Source: CAD feature listing. Evaluate the final solid. Frame: model axes, mm. A direction names the side the tool comes from. Round coordinates to 2 decimals unless told otherwise and drop trailing zeros. Order: outer loops, then holes, each group sorted by start corner. A loop starts at its lowest first (then second) coordinate and runs counter-clockwise, first axis right, second up. Notation, with made-up numbers: (85.5, 64.25) -> (140.5, 64.25) arc R32 ccw to (140.5, 95.25) -> close; hole circle Ø10 at (24, -38). An arc over 180 degrees is marked (long way). Write item = value, one per line. Start each with the question number.
(1) Draft query along X for faces 4 (the face through (-27.25, 28, -8)), 5 (the face through (-22.25, 28.27, -4.83)), 6 (the face through (14.25, 36, 7)). Return one class per face: released by +X, released by -X, zero draft, split by the parting line, or undercut.
(2) Ray query, line 1 (Z direction, x = -24.5, y = 28.5); line 2 (Z direction, x = 24, y = 28); line 3 (Y direction, x = -11, z = -5). Return the intervals inside material, ascending.
(3) Reachability of faces 1 (the face through (-15.55, 38.75, -1.21)), 2 (the face through (-24, 28, -9)), 3 (the face through (4, 36, 9)) from +Z, -Z, +X, -X, +Y, -Y: full face, straight path, thin tool, end or side. Return the list, or none.
(4) Cut plane B-B on z = 0. Return the cut outline in (x, y).
(5) Cut plane C-C on y = 41. Return the cut outline in (x, z).
(6) Cut plane D-D on x = -15. Return the cut outline in (y, z).
(7) Cut plane A-A on x = 24.5. Return the cut outline in (y, z).
(8) Contact query for flat-ended pins moving along their axis: pin 1 Ø1 at (y, z) = (36.5, 8) entering from +X; pin 2 Ø10 at (x, z) = (6.5, 0.5) entering from +Y; pin 3 Ø3.5 at (x, z) = (25, 4) entering from -Y. Output: stop coordinate, or through.
from build123d import *

# Parameters (mm, degrees)
SKETCH1_W            = 40.5
SKETCH1_H            = 20
BOSS_EXTRUDE1_DEPTH  = 35.5
BOSS_EXTRUDE2_DEPTH  = 2
SKETCH3_R            = 6.4
BOSS_EXTRUDE3_DEPTH  = 1
SKETCH4_R            = 5.575
BOSS_EXTRUDE4_DEPTH  = 0.5
BOSS_EXTRUDE5_DEPTH  = 2.5
MIRROR2_COPY_1_DEPTH = 2.5
SKETCH6_R            = 2.5
BOSS_EXTRUDE6_DEPTH  = 5


with BuildPart() as part:
    # Sketch1 → Boss-Extrude1 (new body)
    with BuildSketch(Plane(origin=(0, 0, 0), x_dir=(1, 0, 0), z_dir=(0, 1, 0))):
        Rectangle(SKETCH1_W, SKETCH1_H)
    extrude(amount=BOSS_EXTRUDE1_DEPTH)

    # Sketch2 → Boss-Extrude2 (add)
    with BuildSketch(Plane(origin=(0, 35.5, 0), x_dir=(1, 0, 0), z_dir=(0, 1, 0))):
        with BuildLine():
            Line((-5.75, -9), (14.25, -9))
            Line((14.25, -9), (14.25, -4.8))
            ThreePointArc((14.25, -4.8), (16.65, 0), (14.25, 4.8))
            Line((14.25, 4.8), (14.25, 9))
            Line((14.25, 9), (-5.75, 9))
            ThreePointArc((-5.75, 9), (-20.108898944, 0), (-5.75, -9))
        make_face()
    extrude(amount=BOSS_EXTRUDE2_DEPTH)

    # Sketch3 → Boss-Extrude3 (add)
    with BuildSketch(Plane(origin=(0, 37.5, 0), x_dir=(1, 0, 0), z_dir=(0, 1, 0))):
        with Locations(Location((-10.108898944, 0, 0), (0, 0, 270))):
            Circle(SKETCH3_R)
    extrude(amount=BOSS_EXTRUDE3_DEPTH)

    # Sketch4 → Boss-Extrude4 (add)
    with BuildSketch(Plane(origin=(0, 38.5, 0), x_dir=(1, 0, 0), z_dir=(0, 1, 0))):
        with Locations(Location((-10.108898944, 0, 0), (0, 0, 270))):
            Circle(SKETCH4_R)
    extrude(amount=BOSS_EXTRUDE4_DEPTH)

    # Sketch5 → Boss-Extrude5 (add)
    with BuildSketch(Plane(origin=(0, 29.5, 0), x_dir=(1, 0, 0), z_dir=(0, 1, 0))):
        with BuildLine():
            Line((20.25, 9), (27.25, 9))
            Line((27.25, 9), (27.25, 6.25))
            Line((27.25, 6.25), (26.177050983, 6.25))
            ThreePointArc((26.177050983, 6.25), (22.25, 4.75), (26.177050983, 3.25))
            Line((26.177050983, 3.25), (27.25, 3.25))
            Line((27.25, 3.25), (27.25, 0))
            Line((27.25, 0), (20.25, 0))
            Line((20.25, 0), (20.25, 9))
        make_face()
    boss_extrude5 = extrude(amount=-BOSS_EXTRUDE5_DEPTH)

    # Mirror1: Boss-Extrude5 across plane
    add(boss_extrude5.mirror(Plane(origin=(0, 0, 0), x_dir=(0, 0, 1), z_dir=(1, 0, 0))))

    # Mirror2: Boss-Extrude5 across plane
    add(boss_extrude5.mirror(Plane.XY))

    # Mirror2 copy 1 sketch → Mirror2 copy 1 (add)
    with BuildSketch(Plane(origin=(0, 29.5, 0), x_dir=(-1, 0, 0), z_dir=(0, 1, 0))):
        with BuildLine():
            Line((20.25, 9), (27.25, 9))
            Line((27.25, 9), (27.25, 6.25))
            Line((27.25, 6.25), (26.177050983, 6.25))
            ThreePointArc((26.177050983, 6.25), (22.25, 4.75), (26.177050983, 3.25))
            Line((26.177050983, 3.25), (27.25, 3.25))
            Line((27.25, 3.25), (27.25, 0))
            Line((27.25, 0), (20.25, 0))
            Line((20.25, 0), (20.25, 9))
        make_face()
    extrude(amount=-MIRROR2_COPY_1_DEPTH)

    # Sketch6 → Boss-Extrude6 (add)
    with BuildSketch(Plane(origin=(0, 39, 0), x_dir=(1, 0, 0), z_dir=(0, 1, 0))):
        with Locations(Location((-10.108898944, 0, 0), (0, 0, 270))):
            Circle(SKETCH6_R)
    extrude(amount=BOSS_EXTRUDE6_DEPTH)


solid = part.part
Evaluation:
q1.face_4 = released by -X
q1.face_5 = undercut
q1.face_6 = released by +X
q2.line_1 = -9 to -7, -2.5 to 2.5, 7 to 9
q2.line_2 = -9 to -6.94, -2.56 to 2.56, 6.94 to 9
q2.line_3 = 0 to 39
q3.face_1 = +Y
q3.face_2 = -Z, -X, +Y, -Y
q3.face_3 = +Z, +X, +Y
q4.outline = (-27.25, 27) -> (-20.25, 27) -> (-20.25, 0) -> (20.25, 0) -> (20.25, 27) -> (27.25, 27) -> (27.25, 29.5) -> (20.25, 29.5) -> (20.25, 35.5) -> (16.65, 35.5) -> (16.65, 37.5) -> (-3.71, 37.5) -> (-3.71, 38.5) -> (-4.53, 38.5) -> (-4.53, 39) -> (-7.61, 39) -> (-7.61, 44) -> (-12.61, 44) -> (-12.61, 39) -> (-15.68, 39) -> (-15.68, 38.5) -> (-16.51, 38.5) -> (-16.51, 37.5) -> (-20.11, 37.5) -> (-20.11, 35.5) -> (-20.25, 35.5) -> (-20.25, 29.5) -> (-27.25, 29.5) -> close
q5.outline = circle Ø5 at (-10.11, 0)
q6.outline = (0, -10) -> (35.5, -10) -> (35.5, -8.72) -> (37.5, -8.72) -> (37.5, -4.13) -> (38.5, -4.13) -> (38.5, -2.68) -> (39, -2.68) -> (39, 2.68) -> (38.5, 2.68) -> (38.5, 4.13) -> (37.5, 4.13) -> (37.5, 8.72) -> (35.5, 8.72) -> (35.5, 10) -> (0, 10) -> close
q7.outline = (27, -9) -> (29.5, -9) -> (29.5, -7) -> (27, -7) -> close; (27, -2.5) -> (29.5, -2.5) -> (29.5, 2.5) -> (27, 2.5) -> close; (27, 7) -> (29.5, 7) -> (29.5, 9) -> (27, 9) -> close
q8.pin_1 = 14.25
q8.pin_2 = 37.5
q8.pin_3 = 27
